Verification items for this drawing (mm, ordinates from the low corner). A direction names the side the tool comes from. Coordinates: 2 decimals unless noted, no trailing zeros. Order: outer loops, then holes, each group sorted by start corner. A loop starts at its lowest first (then second) coordinate and runs counter-clockwise, first axis right, second up. Notation, with made-up numbers: M 33,64 L 88,64 A10 cw 88,74 Z; hole C 36,-23 d3. An arc over 180 degrees is marked long. Return JSON: item names as keys, results as strings. Group by question number.
1. Section check A-A, the plane y = 17.75. Record the cut outline in (x, z), plus the area to 3 significant figures.
2. Set-up check for the marked faces 4 and 5: record each of +Z, -Z, +X, -X, +Y, -Y from which the full face is reachable in a straight line by a thin tool's end or side.
3. Mould release check, pull along X, two halves, no side actions. Record for the marked faces 1, 2 and 3: +X half, -X half, draft (parallel to the pull), parting line (faces both ways), or undercut.
4. Section check C-C, the plane x = 4. Record the cut outline in (y, z), plus the area to 3 significant figures.
5. Gauge pin test, flat ends, axial feed: pin 1 (2 mm diameter, centred on y = 7.5, z = 5, fed in from -X); pin 2 (5 mm diameter, centred on x = 54.5, z = 6.5, fed in from +Y); pin 3 (7 mm diameter, centred on x = 4, z = 7.5, fed in from +Y). Record the tip position at first contact, or that the pin passes through.
6. Section check D-D, the plane x = 35. Record the cut outline in (y, z), plus the area to 3 significant figures.
7. Section check B-B, the plane z = 14. Record the cut outline in (x, y).
8. Material ranges on line 1 along Z through (x, y) = (66, 7.8); line 2 along X through (y, z) = (2.75, 7.5); line 3 along Z through (x, y) = (4, 4.75), recorded low to high.
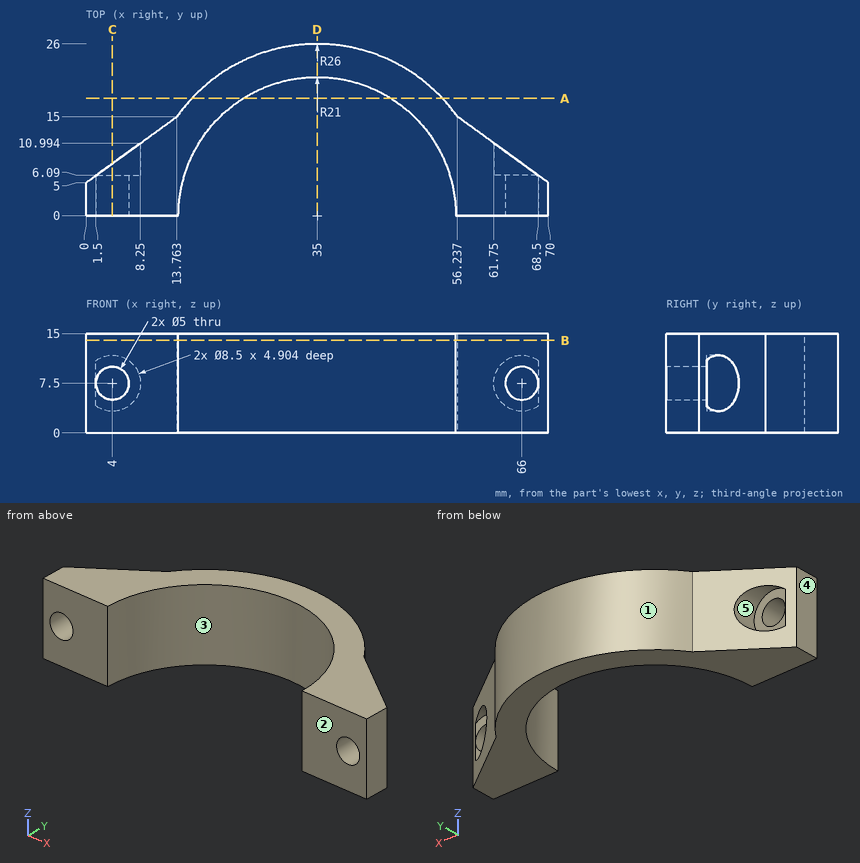
Answers follow:
{
 "1": {"outline": "M 16,0 L 23.78,0 L 23.78,15 L 16,15 Z; M 46.22,0 L 54,0 L 54,15 L 46.22,15 Z", "area": "233 mm^2"},
 "2": {"face 4": "+Z, -Z, -X, +Y, -Y", "face 5": "+Y"},
 "3": {"face 1": "parting line", "face 2": "draft", "face 3": "undercut"},
 "4": {"outline": "M 0,0 L 7.91,0 L 7.91,3.25 L 6.09,3.25 L 6.09,5 L 0,5 Z; M 0,10 L 6.09,10 L 6.09,11.75 L 7.91,11.75 L 7.91,15 L 0,15 Z", "area": "72.7 mm^2"},
 "5": {"pin 1": "x = 6.41", "pin 2": "y = 19.67", "pin 3": "y = 6.09"},
 "6": {"outline": "M 21,0 L 26,0 L 26,15 L 21,15 Z", "area": "75.0 mm^2"},
 "7": {"outline": "M 0,0 L 14,0 A21 cw 56,0 L 70,0 L 70,5 L 56.24,15 A26 ccw 13.76,15 L 0,5 Z"},
 "8": {"line 1": "0 to 3.25, 11.75 to 15", "line 2": "0 to 1.5, 6.5 to 14.18, 55.82 to 63.5, 68.5 to 70", "line 3": "0 to 5, 10 to 15"}
}
